from build123d import *

# Parameters (mm, degrees)
F0_W      = 36
F0_H      = 45
F0_R      = 5.5
F1_DEPTH  = 1.5
F2_W      = 19
F2_H      = 24
F2_R      = 5.5
F3_DEPTH  = 12
F4_W      = 36
F4_H      = 45
F4_W_2    = 19
F4_H_2    = 24
F4_R      = 5.5
F5_DEPTH  = 1.5
F6_R      = 0.75
F7_DEPTH  = 2.5
F8_W      = 36
F8_H      = 4
F9_DEPTH  = 1.5
F10_W     = 36
F10_H     = 4
F11_DEPTH = 1.5
F12_R     = 5
F13_R     = 3


with BuildPart() as f1:
    # F0 (on Front) → F1 (new body)
    with BuildSketch(Plane.XZ):
        Rectangle(F0_W, F0_H)
        Circle(F0_R, mode=Mode.SUBTRACT)
    extrude(amount=F1_DEPTH)

    # F2 (on face) → F3 (join)
    with BuildSketch(Plane.XZ.offset(1.5)):
        Rectangle(F2_W, F2_H)
        Circle(F2_R, mode=Mode.SUBTRACT)
    extrude(amount=F3_DEPTH)

    # F4 (on face) → F5 (join)
    with BuildSketch(Plane.XZ.offset(13.5)):
        Rectangle(F4_W, F4_H)
        Rectangle(F4_W_2, F4_H_2, mode=Mode.SUBTRACT)
        Rectangle(F4_W_2, F4_H_2)
        Circle(F4_R, mode=Mode.SUBTRACT)
    extrude(amount=-F5_DEPTH)

    # F6 (on face) → F7 (cut)
    with BuildSketch(Plane.XZ.offset(13.5)):
        with Locations((-7.9445969313, -10.7102040201)):
            Circle(F6_R)
    extrude(amount=-F7_DEPTH, mode=Mode.SUBTRACT)

    # F8 (on face) → F9 (join)
    with BuildSketch(Plane.XZ.offset(13.5)):
        with Locations((0, 24.5)):
            Rectangle(F8_W, F8_H)
    extrude(amount=-F9_DEPTH)

    # F10 (on face) → F11 (join)
    with BuildSketch(Plane(origin=(0, 0, 0), x_dir=(-1, 0, 0), z_dir=(0, 1, 0))):
        with Locations((0, 24.5)):
            Rectangle(F10_W, F10_H)
    extrude(amount=-F11_DEPTH)

    # F12
    f12_edges = [f1.edges().sort_by_distance(p)[0] for p in [
        (18, -12.75, 26.5),
        (18, -0.75, 26.5),
        (18, -0.75, -22.5),
        (18, -12.75, -22.5),
        (-18, -0.75, -22.5),
        (-18, -12.75, -22.5),
        (-18, -0.75, 26.5),
        (-18, -12.75, 26.5),
    ]]
    fillet(f12_edges, radius=F12_R)

    # F13
    f13_edges = [f1.edges().sort_by_distance(p)[0] for p in [
        (-9.5, -6.75, 12),
        (9.5, -6.75, 12),
        (9.5, -6.75, -12),
        (-9.5, -6.75, -12),
    ]]
    fillet(f13_edges, radius=F13_R)


solid = f1.part
Can you work these out from the model? Positions are in its coordinate system, mm. A direction names the side the tool comes from. Round coordinates to 2 decimals unless told otherwise and drop trailing zeros. Order: outer loops, then holes, each group sorted by start corner. A loop starts at its lowest first (then second) coordinate and runs counter-clockwise, first axis right, second up. Notation, with made-up numbers: (58, 42) - (73, 42) arc R24 ccw to (73, 80) - close; hole circle Ø9 at (-4, 44). An arc over 180 degrees is marked (long way). Answer in a Markdown table with one row per item.
(1) Suppose I cut it at B-B, the plane x = 0. Please give me the cut outline in (y, z).
From the geometry:
| item | result |
|---|---|
| outline | (-13.5, -22.5) - (-12, -22.5) - (-12, -12) - (-1.5, -12) - (-1.5, -22.5) - (0, -22.5) - (0, -5.5) - (-13.5, -5.5) - close; (-13.5, 5.5) - (0, 5.5) - (0, 26.5) - (-1.5, 26.5) - (-1.5, 12) - (-12, 12) - (-12, 26.5) - (-13.5, 26.5) - close |
(2) Please list where these lines run through material, in increasing order: L1, parallel to Z at x = 0, y = -6; L2, parallel to Y at x = 13, z = 8; L3, parallel to Z at x = -5, y = -3.5. Write a range as from..to.
From the geometry:
| item | result |
|---|---|
| L1 | z = -12..-5.5, 5.5..12 |
| L2 | y = -13.5..-12, -1.5..0 |
| L3 | z = -12..-2.29, 2.29..12 |
(3) Suppose I cut it at D-D, the plane z = 0. Please give me the cut outline in (x, y).
From the geometry:
| item | result |
|---|---|
| outline | (-18, -13.5) - (-5.5, -13.5) - (-5.5, 0) - (-18, 0) - (-18, -1.5) - (-9.5, -1.5) - (-9.5, -12) - (-18, -12) - close; (5.5, -13.5) - (18, -13.5) - (18, -12) - (9.5, -12) - (9.5, -1.5) - (18, -1.5) - (18, 0) - (5.5, 0) - close |
(4) Suppose I cut it at A-A, the plane y = -4.25. Please give me the cut outline in (x, z), plus the area to 3 significant figures.
From the geometry:
| item | result |
|---|---|
| outline | (-9.5, -9) arc R3 ccw to (-6.5, -12) - (6.5, -12) arc R3 ccw to (9.5, -9) - (9.5, 9) arc R3 ccw to (6.5, 12) - (-6.5, 12) arc R3 ccw to (-9.5, 9) - close; hole circle Ø11 at (0, 0) |
| area | 353 mm2 |
(5) Which directions (+Z, -Z, +X, -X, +Y, -Y) give clear straight access to the entire face, cutting with the end or side of a thin tool? Please do faces 3 (the face through (-8.64, -6.82, -11.1)), 4 (the face through (0, -7, -12)), 5 (the face through (-8.54, -12.268, -11.167)), 6 (the face through (0, -12, 13)), 7 (the face through (-9.5, -7, 0)).
From the geometry:
| item | result |
|---|---|
| face 3 | -Z, -X |
| face 4 | -Z, +X, -X |
| face 5 | -Y |
| face 6 | none |
| face 7 | +Z, -Z, -X |
(6) Suppose I cut it at C-C, the plane z = -16.5. Please give me the cut outline in (x, y), plus the area to 3 significant figures.
From the geometry:
| item | result |
|---|---|
| outline | (-18, -13.5) - (18, -13.5) - (18, -12) - (-18, -12) - close; (-18, -1.5) - (18, -1.5) - (18, 0) - (-18, 0) - close |
| area | 108 mm2 |
(7) For P1, Ø1.4, axis at x = -7.94, z = -10.71, coming from the -Y side; P2, Ø5, axis at y = -7.5, z = 1, coming from the -X side; P3, Ø5, axis at y = -8, z = 16, coming from the +X side; P4, Ø3, axis at y = -4, z = 9.5, coming from the +X side, each with a flat end and sliding along its axis, tell me the tip position at first contact or that it passes through.
From the geometry:
| item | result |
|---|---|
| P1 | stops at y = -11 |
| P2 | stops at x = -9.5 |
| P3 | passes through |
| P4 | stops at x = 9.5 |
(8) If we mould it in two halves opening along Y, with no side actions, what happens to faces 1 (the face through (9.5, -7, 0)), 2 (the face through (16.57, -0.76, 25))? For each: released by +Y, released by -Y, zero draft, split by the parting line, or undercut.
From the geometry:
| item | result |
|---|---|
| face 1 | undercut |
| face 2 | zero draft |
